Geometry: see drawing. Coordinates: mm, zero at the bounding-box minimum. A direction names the side the tool comes from. Round coordinates to 2 decimals unless told otherwise and drop trailing zeros. Loops run counter-clockwise (first coordinate to the right, second up) from the corner with the lowest first, then second, coordinate; pieces in that order, holes last. Notation, with made-up numbers: (-3.5, 41) -> (30.5, 41) arc R32 cw to (30.5, 70) -> close; hole circle Ø3 at (55.25, 27). An arc over 180 degrees is marked (long way). Write item = value, one per line.
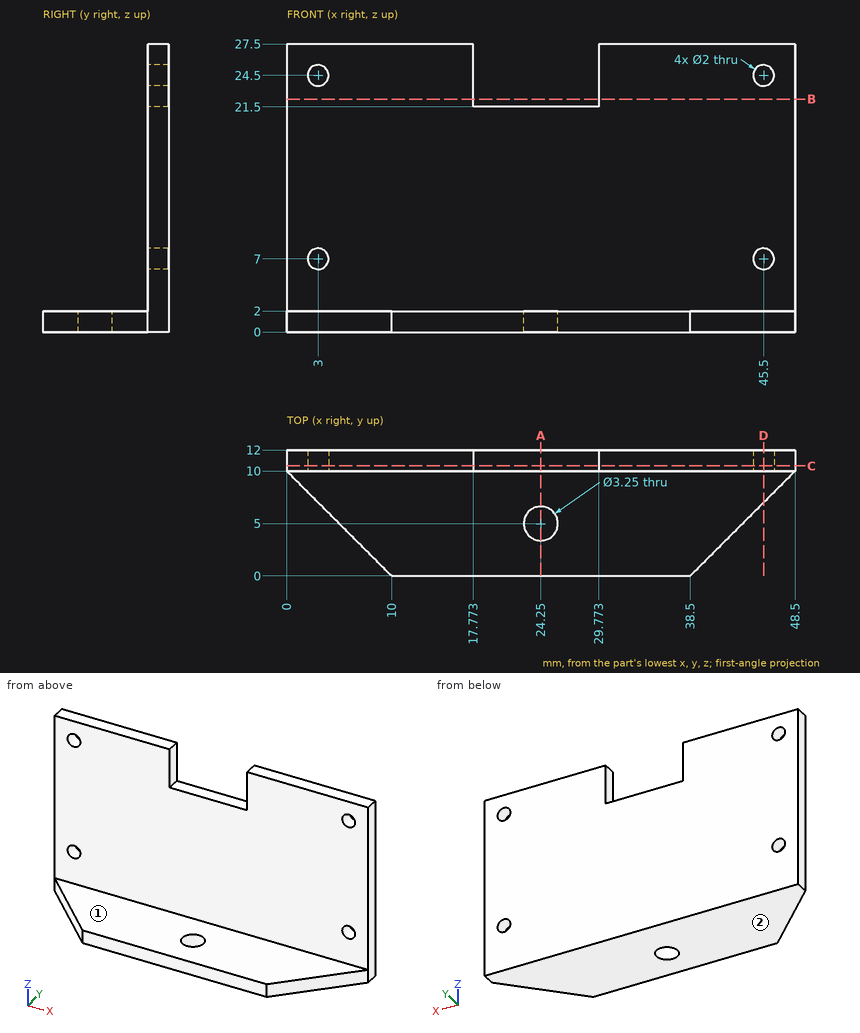
1. Section query C-C (y = 10.5). Return the cut outline in (x, z).
Evaluation:
outline = (0, 0) -> (48.5, 0) -> (48.5, 27.5) -> (29.77, 27.5) -> (29.77, 21.5) -> (17.77, 21.5) -> (17.77, 27.5) -> (0, 27.5) -> close; hole circle Ø2 at (3, 7); hole circle Ø2 at (3, 24.5); hole circle Ø2 at (45.5, 7); hole circle Ø2 at (45.5, 24.5)
2. Section query D-D (x = 45.5). Return the cut outline in (y, z), then the cut area to 3 significant figures.
Evaluation:
outline = (7, 0) -> (12, 0) -> (12, 6) -> (10, 6) -> (10, 2) -> (7, 2) -> close; (10, 8) -> (12, 8) -> (12, 23.5) -> (10, 23.5) -> close; (10, 25.5) -> (12, 25.5) -> (12, 27.5) -> (10, 27.5) -> close
area = 53.0 mm²
3. Section query A-A (x = 24.25). Return the cut outline in (y, z) (3 decimals).
Evaluation:
outline = (0, 0) -> (3.375, 0) -> (3.375, 2) -> (0, 2) -> close; (6.625, 0) -> (12, 0) -> (12, 21.5) -> (10, 21.5) -> (10, 2) -> (6.625, 2) -> close
4. Set-up query: the marked faces 1 and 2. Return all of +Z, -Z, +X, -X, +Y, -Y with unobstructed straight access to the full face (end or side cutting, diameter ignored); none if empty.
Evaluation:
face_1 = +Z, +X, -X, -Y
face_2 = -Z, +X, -X, +Y, -Y
5. Contact query for flat-ended pins moving along their axis: pin 1 Ø2.5 at (x, z) = (3, 7) entering from -Y; pin 2 Ø5 at (x, y) = (42, 3) entering from -Z; pin 3 Ø4 at (x, y) = (41.5, 6.5) entering from +Z; pin 4 Ø1 at (x, y) = (22, 11) entering from +Z. Output: stop coordinate, or through.
Evaluation:
pin_1 = 10
pin_2 = 0
pin_3 = 2
pin_4 = 21.5
6. Section query B-B (z = 22.25). Return the cut outline in (x, y).
Evaluation:
outline = (0, 10) -> (17.77, 10) -> (17.77, 12) -> (0, 12) -> close; (29.77, 10) -> (48.5, 10) -> (48.5, 12) -> (29.77, 12) -> close
7. Line query: probe 1 along X at (y, z) = (11.15, 24.5); probe 2 along Z at (x, y) = (45.5, 10.95); probe 3 along X at (y, z) = (10.55, 7). Output: solid intervals per line, ascending. Write a range as from..to.
Evaluation:
probe_1 = 0..2, 4..17.77, 29.77..44.5, 46.5..48.5
probe_2 = 0..6, 8..23.5, 25.5..27.5
probe_3 = 0..2, 4..44.5, 46.5..48.5
